from build123d import *

# Parameters (mm, degrees)
F1_DEPTH = 2114


with BuildPart() as f1:
    # F0 (on Top) → F1 (new body)
    with BuildSketch(Plane.XY):
        with BuildLine():
            Line((-45, 0), (0, 0))
            Line((0, 0), (0, 6))
            Line((0, 6), (-39, 6))
            ThreePointArc((-39, 6), (-42.535534, 7.464466), (-44, 11))
            Line((-44, 11), (-44, 146))
            ThreePointArc((-44, 146), (-42.535534, 149.535534), (-39, 151))
            Line((-39, 151), (-1, 151))
            ThreePointArc((-1, 151), (2.535534, 149.535534), (4, 146))
            Line((4, 146), (4, 121))
            ThreePointArc((4, 121), (5.464466, 117.464466), (9, 116))
            Line((9, 116), (55, 116))
            Line((55, 116), (55, 122))
            Line((55, 122), (15, 122))
            ThreePointArc((15, 122), (11.464466, 123.464466), (10, 127))
            Line((10, 127), (10, 152))
            ThreePointArc((10, 152), (8.535534, 155.535534), (5, 157))
            Line((5, 157), (-45, 157))
            ThreePointArc((-45, 157), (-48.535534, 155.535534), (-50, 152))
            Line((-50, 152), (-50, 5))
            ThreePointArc((-50, 5), (-48.535534, 1.464466), (-45, 0))
        make_face()
    extrude(amount=F1_DEPTH)


solid = f1.part
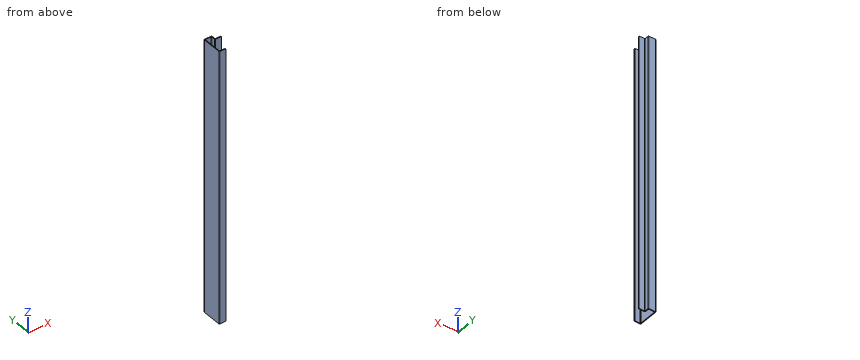
Geometry: final body of the model. Coordinates: model frame, mm. Give positions to 0.01 mm unless a question says otherwise; leave off trailing zeros. Write each loop counter-clockwise with the first axis right and the second up, starting at its lowest first coordinate (ties: lowest second). Pieces come first, ordered by that corner, then holes. Notation, with made-up numbers: (87, -7.5) -> (140, -7.5) arc R25 cw to (140, 20.5) -> close; hole circle Ø5 at (8, 6). An arc over 180 degrees is marked (long way). Answer in a Markdown table with one row per item.
(1) Ray query, line 1 along X through (y, z) = (125.5, 1050); line 2 along Y through (x, z) = (-13, 297.5); line 3 along X through (y, z) = (139, 1783). Return the intervals inside material, ascending. Write a range as [from, to].
Answers below:
| item | result |
|---|---|
| line 1 | [-50, -44], [4, 10.23] |
| line 2 | [0, 6], [151, 157] |
| line 3 | [-50, -44], [4, 10] |
(2) Section query B-B on z = 403. Return loops of the section in (x, y).
Answers below:
| item | result |
|---|---|
| outline | (-50, 5) arc R5 ccw to (-45, 0) -> (0, 0) -> (0, 6) -> (-39, 6) arc R5 cw to (-44, 11) -> (-44, 146) arc R5 cw to (-39, 151) -> (-1, 151) arc R5 cw to (4, 146) -> (4, 121) arc R5 ccw to (9, 116) -> (55, 116) -> (55, 122) -> (15, 122) arc R5 cw to (10, 127) -> (10, 152) arc R5 ccw to (5, 157) -> (-45, 157) arc R5 ccw to (-50, 152) -> close |
(3) Pin query (flat end, axial travel): pin 1 (4 mm diameter, centred on x = 26.5, z = 1515, fed in from +Y); pin 2 (20 mm diameter, centred on y = 141.5, z = 1396, fed in from +X); pin 3 (1.8 mm diameter, centred on y = 3, z = 1517, fed in from +X). Return the tip coordinate at first contact, or that it passes through.
Answers below:
| item | result |
|---|---|
| pin 1 | y = 122 |
| pin 2 | x = 10 |
| pin 3 | x = 0 |
(4) Section query A-A on x = -22. Return loops of the section in (y, z), then the cut area to 3 significant figures.
Answers below:
| item | result |
|---|---|
| outline | (0, 0) -> (6, 0) -> (6, 2114) -> (0, 2114) -> close; (151, 0) -> (157, 0) -> (157, 2114) -> (151, 2114) -> close |
| area | 25,400 mm^2 |
(5) Section query C-C on y = 28. Return loops of the section in (x, z), then the cut area to 3 significant figures.
Answers below:
| item | result |
|---|---|
| outline | (-50, 0) -> (-44, 0) -> (-44, 2114) -> (-50, 2114) -> close |
| area | 12,700 mm^2 |
